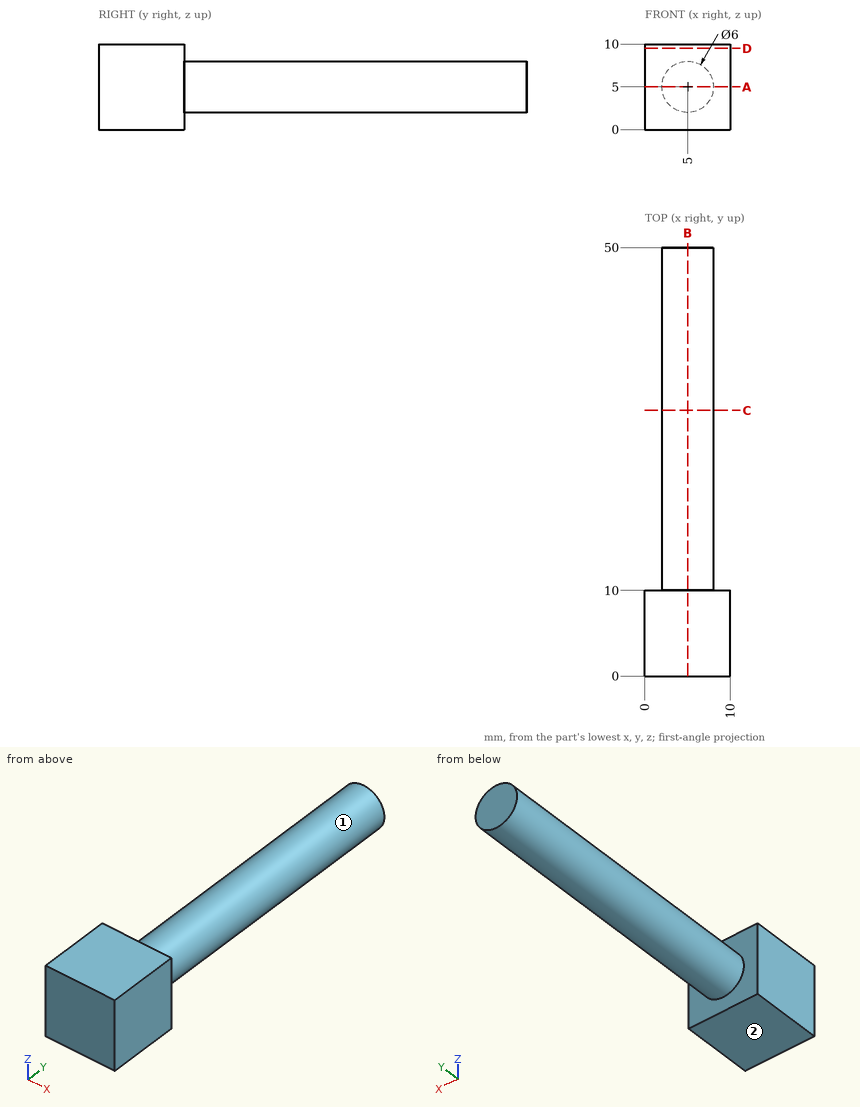
Geometry check sheet. Reference: drawing and pictorial views, mm from the part's lowest x, y, z. A direction names the side the tool comes from. Round coordinates to 2 decimals unless told otherwise and drop trailing zeros. Loops run counter-clockwise (first coordinate to the right, second up) from the corner with the lowest first, then second, coordinate; pieces in that order, holes last.
1. Sectioned sample at A-A on z = 5. Record the boundary of the cut face in (x, y), and give its area (3 significant figures).
2. Gauge pin test, flat ends, axial feed: pin 1 Ø5 at (y, z) = (29.5, 3) entering from +X; pin 2 Ø4 at (y, z) = (19, 7) entering from -X. Record the tip position at first contact, or that the pin passes through.
3. Set-up check for the marked faces 1 and 2: record each of +Z, -Z, +X, -X, +Y, -Y from which the full face is reachable in a straight line by a thin tool's end or side.
4. Sectioned sample at D-D on z = 9.5. Record the boundary of the cut face in (x, y), and give its area (3 significant figures).
5. Scan lines: probe 1 along Y at (x, z) = (1.25, 7); probe 2 along Z at (x, y) = (5.25, 42.5). Record each from-to range of solid material in increasing order.
6. Sectioned sample at B-B on x = 5. Record the boundary of the cut face in (y, z).
7. Sectioned sample at C-C on y = 31. Record the boundary of the cut face in (x, z), and give its area (3 significant figures).
Recorded:
1. outline: (0, 0) - (10, 0) - (10, 10) - (8, 10) - (8, 50) - (2, 50) - (2, 10) - (0, 10) - close
1. area: 340 mm2
2. pin 1: stops at x = 8
2. pin 2: stops at x = 2
3. face 1: +Y
3. face 2: -Z, +X, -X, +Y, -Y
4. outline: (0, 0) - (10, 0) - (10, 10) - (0, 10) - close
4. area: 100 mm2
5. probe 1: y = 0 to 10
5. probe 2: z = 2.01 to 7.99
6. outline: (0, 0) - (10, 0) - (10, 2) - (50, 2) - (50, 8) - (10, 8) - (10, 10) - (0, 10) - close
7. outline: circle Ø6 at (5, 5)
7. area: 28.3 mm2
